Geometry check sheet. Reference: the model listing, model coordinates, mm. Face numbers are marked on the shaded views. Round coordinates to 2 decimals unless told otherwise and drop trailing zeros. Order: outer loops, then holes, each group sorted by start corner. A loop starts at its lowest first (then second) coordinate and runs counter-clockwise, first axis right, second up. Notation, with made-up numbers: (11.25, 6) - (19.25, 6) arc R34 ccw to (19.25, 38) - close; hole circle Ø11 at (14.25, 88.25). An arc over 180 degrees is marked (long way). Use a Markdown table: item, result. Add a question column.
(1) Thickness scan on line 1 along X through (y, z) = (0, 6.5); line 2 along Z through (x, y) = (15, -23); line 3 along Y through (x, z) = (39, 1.5). Record the ranges inside material, lowest first. Write a range as [from, to].
(2) Section check A-A on y = 31. Record the boundary of the cut face in (x, z), then the cut area to 3 significant figures.
(3) Mould release check, pull along Y, two halves, no side actions. Record for the marked faces 1, 2 and 3: released by +Y, released by -Y, zero draft, split by the parting line, or undercut.
(4) Gauge pin test, flat ends, axial feed: P1, Ø1.5, axis at y = 26.5, z = 0.5, coming from the -X side; P2, Ø4, axis at x = 15, z = 4.5, coming from the -Y side; P3, Ø3, axis at y = 4.5, z = 4.5, coming from the +X side. Record the tip position at first contact, or that the pin passes through.
(5) Section check C-C on z = 3.75. Record the boundary of the cut face in (x, y).
(6) Section check B-B on x = 14. Record the boundary of the cut face in (y, z).
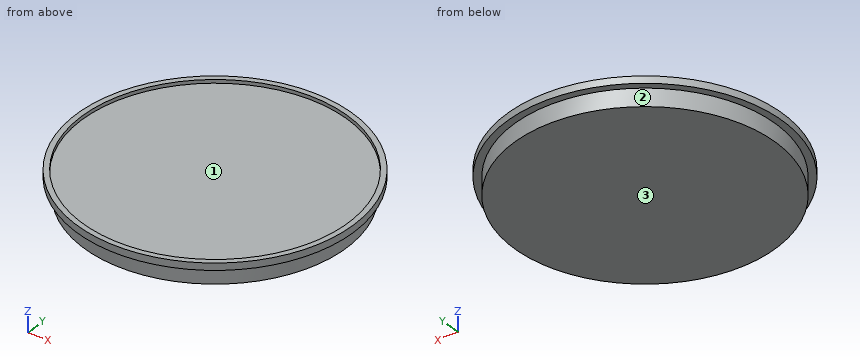
Autodesk Inventor part; units mm, degrees
ref_plane "工作平面1" through (38.9425, 38.9425, 0) normal (1, 0, 0) x (0, 1, 0)
ref_plane "XZ Plane" through (0, 0, 0) normal (0, 1, 0) x (-1, 0, 0)
ref_plane "XY Plane" through (0, 0, 0) normal (0, 0, 1) x (1, 0, 0)
sketch "草圖1" plane through (6.7908, 20.3797, 0) normal (0, 0, -1) x (-1, 0, 0)
  circle A0 centre (-32.1517, 18.5628) radius 37.1256
  point P0 (6.7908, -20.3797)
ref_plane "工作平面1" through (38.9425, 38.9425, 0) normal (1, 0, 0) x (0, 1, 0)
sketch "草圖2" plane through (38.9425, 38.9425, 0) normal (1, 0, 0) x (0, 1, 0)
  line L0 (-38.9425, 0) -> (-38.9425, 6)
  line L1 (-38.9425, 6) -> (-76.4425, 6)
  line L2 (-76.4425, 6) -> (-76.4425, 7)
  line L3 (-76.4425, 7) -> (-77.9425, 7)
  line L4 (-77.9425, 7) -> (-77.9425, 5)
  line L5 (-77.9425, 5) -> (-75.9425, 5)
  line L6 (-75.9425, 5) -> (-75.9425, 0)
  line L7 (-75.9425, 0) -> (-38.9425, 0)
  dimension "d0" = 74
  dimension "d1" = 78
  dimension "d4" = 75
  dimension "d7" = 7
  dimension "d8" = 5
  dimension "d9" = 6
revolve "迴轉1" add sketch "草圖2" angle 360 about axis through (38.9425, 0, 0) along (0, 0, 1)
properties part number "下" material "SS41"
Check sheet entries:
| question | item | result |
|---|---|---|
| 1 | line 1 | x = [-0.06, 1.44], [76.44, 77.94] |
| 1 | line 2 | z = [0, 6] |
| 1 | line 3 | y = [-37, 37] |
| 2 | outline | (15.28, 5) - (18.74, 5) - (18.74, 0) - (59.14, 0) - (59.14, 5) - (62.61, 5) - (62.61, 7) - (60.04, 7) - (60.04, 6) - (17.84, 6) - (17.84, 7) - (15.28, 7) - close |
| 2 | area | 254 mm2 |
| 3 | face 1 | undercut |
| 3 | face 2 | split by the parting line |
| 3 | face 3 | zero draft |
| 4 | P1 | stops at x = 12.37 |
| 4 | P2 | stops at y = -32.2 |
| 4 | P3 | stops at x = 77.82 |
| 5 | outline | circle Ø74 at (38.94, 0) |
| 6 | outline | (-29.98, 5) - (-27.33, 5) - (-27.33, 0) - (27.33, 0) - (27.33, 5) - (29.98, 5) - (29.98, 7) - (28, 7) - (28, 6) - (-28, 6) - (-28, 7) - (-29.98, 7) - close |
